Input: part model. Units: mm. Frame: model coordinates. Round coordinates to 2 decimals unless told otherwise and drop trailing zeros. Loops run counter-clockwise (first coordinate to the right, second up) from the corner with the lowest first, then second, coordinate; pieces in that order, holes last. Notation, with made-up numbers: M 56.5,18 L 79.5,18 A24 ccw 79.5,52 Z; hole C 79,-38 d11. An arc over 180 degrees is marked long. Put each result on its own line as item: value. Start each with the question number.
1) Section A-A on z = 3.75. Output: boundary loops of the cut face in (x, y), plus the area to 3 significant figures.
2) Draft query along Z for faces 1 (the face through (5.92, -2.01, 4.99)), 2 (the face through (0, 0, 0)). Return one class per face: +Z half, -Z half, draft (parallel to the pull), parting line (faces both ways), or undercut.
3) Section D-D on y = -1. Output: boundary loops of the cut face in (x, z), plus the area to 3 significant figures.
4) Line query: probe 1 along Z at (x, y) = (8, 4); probe 2 along Z at (x, y) = (2.5, 4.75). Output: solid intervals per line, ascending.
5) Pin query (flat end, axial travel): pin 1 (1.5 mm diameter, centred on x = 2, z = 4.5, fed in from +Y); pin 2 (1.5 mm diameter, centred on x = 7.5, y = -3, fed in from -Z). Return the tip coordinate at first contact, or that it passes through.
6) Section C-C on z = -4.75. Output: boundary loops of the cut face in (x, y), plus the area to 3 significant figures.
from build123d import *

# Parameters (mm, degrees)
BASPROSKE_W         = 12
BASPROSKE_H         = 6.3
TOOTHCUT_DEPTH      = 15.945902448
TEETHCUTS_COUNT     = 12
TEETHCUTS_ANGLE     = 330
BORE_DEPTH          = 50.0000508
BOSS_EXTRUDE1_DEPTH = 12


with BuildPart() as part:
    # BasProSke → Base-Revolve (revolve)
    with BuildSketch(Plane(origin=(0, 0, 0), x_dir=(1, 0, 0), z_dir=(0, 1, 0)), mode=Mode.PRIVATE) as base_revolve_sk:
        with Locations((6, 3.15)):
            Rectangle(BASPROSKE_W, BASPROSKE_H)
    revolve(base_revolve_sk.sketch.rotate(Axis((-10, 0, 0), (1, 0, 0)), 180), axis=Axis((-10, 0, 0), (1, 0, 0)))

    # TooCutSke → ToothCut (cut, through all)
    with BuildSketch(Plane(origin=(0, 0, 0), x_dir=(0, 0, -1), z_dir=(1, 0, 0))):
        with BuildLine():
            ThreePointArc((0.505712998, 4.243975773), (0, 4.274), (-0.505712998, 4.243975773))
            ThreePointArc((-0.505712998, 4.243975773), (-0.754225381, 5.326869831), (-1.508135905, 6.142980649))
            ThreePointArc((-1.508135905, 6.142980649), (0, 6.3254), (1.508135905, 6.142980649))
            ThreePointArc((1.508135905, 6.142980649), (0.754225381, 5.326869831), (0.505712998, 4.243975773))
        make_face()
    toothcut = extrude(amount=TOOTHCUT_DEPTH, mode=Mode.SUBTRACT)

    # TeethCuts: ToothCut ×12 about axis
    teethcuts_axis = Axis((-10, 0, 0), (1, 0, 0))
    for i in range(1, TEETHCUTS_COUNT):
        add(toothcut.rotate(teethcuts_axis, i * TEETHCUTS_ANGLE / (TEETHCUTS_COUNT - 1)), mode=Mode.SUBTRACT)

    # BorSke → Bore (cut, symmetric)
    with BuildSketch(Plane(origin=(0, 0, 0), x_dir=(0, 0, -1), z_dir=(1, 0, 0))):
        with BuildLine():
            Line((-1.5, 2), (1.5, 2))
            ThreePointArc((1.5, 2), (0, -2.5), (-1.5, 2))
        make_face()
    extrude(amount=BORE_DEPTH, both=True, mode=Mode.SUBTRACT)

    # Sketch1 → Boss-Extrude1 (add)
    with BuildSketch(Plane(origin=(12, 0, 0), x_dir=(0, 0, -1), z_dir=(1, 0, 0))):
        with BuildLine():
            Line((1.5, 2), (-1.5, 2))
            ThreePointArc((-1.5, 2), (0, -2.5), (1.5, 2))
        make_face()
    extrude(amount=-BOSS_EXTRUDE1_DEPTH)


solid = part.part
Geometry results:
1. outline: M 0,-4.45 L 12,-4.45 L 12,-2.77 L 0,-2.77 Z; M 0,-2.05 L 12,-2.05 L 12,2.05 L 0,2.05 Z; M 0,2.77 L 12,2.77 L 12,4.45 L 0,4.45 Z
1. area: 89.3 mm²
2. face 1: undercut
2. face 2: draft
3. outline: M 0,-5.7 L 12,-5.7 L 12,5.7 L 0,5.7 Z
3. area: 137 mm²
4. probe 1: z = -4.52 to -3.01, -1.73 to 1.73, 3.01 to 4.52
4. probe 2: z = -1.99 to -0.55, 0.55 to 1.99
5. pin 1: stops at y = 4.56
5. pin 2: stops at z = -4.45
6. outline: M 0,-1.99 L 12,-1.99 L 12,-0.55 L 0,-0.55 Z; M 0,0.55 L 12,0.55 L 12,1.99 L 0,1.99 Z
6. area: 34.6 mm²
